Geometry check sheet. Reference: the model listing, model coordinates, mm. Face numbers are marked on the shaded views. A direction names the side the tool comes from. Give positions to 0.01 mm unless a question says otherwise; leave off trailing zeros. Write each loop counter-clockwise with the first axis right and the second up, starting at its lowest first coordinate (ties: lowest second). Pieces come first, ordered by that corner, then holes. Notation, with made-up numbers: M -8.75,25.5 L -3.75,25.5 A21 cw -3.75,40.5 Z; hole C 69.5,-16.5 d9. An arc over 180 degrees is marked long. One line per item, written item: value. Start each with the question number.
1. Gauge pin test, flat ends, axial feed: pin 1 (1.5 mm diameter, centred on x = 3.5, z = 2.5, fed in from -Y); pin 2 (0.8 mm diameter, centred on x = 16, y = 38.5, fed in from +Z); pin 3 (5 mm diameter, centred on x = 9.5, z = 4.5, fed in from -Y); pin 4 (1 mm diameter, centred on x = 8.5, z = 5, fed in from -Y). Record the tip position at first contact, or that the pin passes through.
2. Scan lines: line 1 (X direction, y = 23, z = 5.25); line 2 (Z direction, x = 24.75, y = 4.5); line 3 (Y direction, x = 8.25, z = 7.75). Record each from-to range of solid material in increasing order.
3. Release check for a two-part mould opening along Y. For the marked faces 3, 4 and 5 record: pulls with the +Y half, pulls with the -Y half, needs draft (parallel to the pull), parting line crosses it, or undercut.
4. Cross-section at A-A on x = 17.75. Record the cut outline in (y, z), then the cut area to 3 significant figures.
5. Cross-section at D-D on y = 19. Record the cut outline in (x, z), then the cut area to 3 significant figures.
6. Cross-section at B-B on y = 7.5. Record the cut outline in (x, z), then the cut area to 3 significant figures.
7. Tool access check on the marked faces 1 and 2. Record the directions out of +Z, -Z, +X, -X, +Y, -Y that give a thin tool (end or side, any length) a straight path to the whole face; none if there is none.
8. Cross-section at C-C on z = 3.75. Record the cut outline in (x, y), then the cut area to 3 significant figures.
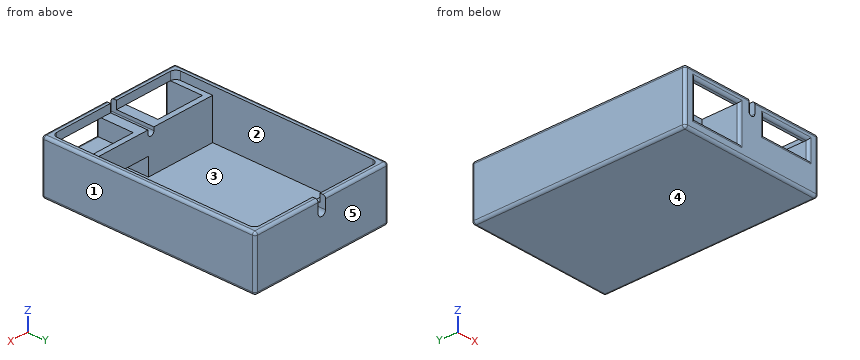
from build123d import *

# Parameters (mm, degrees)
SKETCH_2_W           = 27
SKETCH_2_H           = 40
EXTRUDE_1_DEPTH      = 10
CUT_EXTRUDE_1_DEPTH  = 1.5
CUT_EXTRUDE_2_DEPTH  = 7.5
SKETCH_9_W           = 9
SKETCH_9_H           = 4.718038217
CUT_EXTRUDE_8_DEPTH  = 3.2
SKETCH_9_3_W         = 9
SKETCH_9_3_H         = 4.718038217
CUT_EXTRUDE_9_DEPTH  = 6.5
SKETCH_12_W          = 12
SKETCH_12_H          = 3.3
CUT_EXTRUDE_10_DEPTH = 7
SKETCH_13_W          = 9
SKETCH_13_H          = 6.5
SKETCH_13_H_2        = 3.2
CUT_EXTRUDE_11_DEPTH = 3.281961783
CUT_EXTRUDE_12_REACH = 42
SKETCH_14_W          = 1.2
SKETCH_14_H          = 2.1
SKETCH_16_2_W        = 7
SKETCH_16_2_H        = 2.5
EXTRUDE_3_DEPTH      = 1
SKETCH_16_W          = 7
SKETCH_16_H          = 2.5
EXTRUDE_2_DEPTH      = 1
CUT_EXTRUDE_14_DEPTH = 2
FILLET_1_R           = 0.5


with BuildPart() as part:
    # Sketch 2 → Extrude 1 (new body)
    with BuildSketch(Plane.XY):
        with Locations((13.5, 20)):
            Rectangle(SKETCH_2_W, SKETCH_2_H)
    extrude(amount=EXTRUDE_1_DEPTH)

    # Sketch 3 → Cut-Extrude 1 (cut)
    with BuildSketch(Plane.XY.offset(10)):
        with BuildLine():
            Line((1, 38), (1, 2))
            ThreePointArc((1, 2), (1.292893219, 1.292893219), (2, 1))
            Line((2, 1), (25, 1))
            ThreePointArc((25, 1), (25.707106781, 1.292893219), (26, 2))
            Line((26, 2), (26, 38))
            ThreePointArc((26, 38), (25.707106781, 38.707106781), (25, 39))
            Line((25, 39), (2, 39))
            ThreePointArc((2, 39), (1.292893219, 38.707106781), (1, 38))
        make_face()
    extrude(amount=-CUT_EXTRUDE_1_DEPTH, mode=Mode.SUBTRACT)

    # Sketch 5 → Cut-Extrude 2 (cut)
    with BuildSketch(Plane.XY.offset(8.5)):
        with BuildLine():
            Line((2, 39), (25, 39))
            ThreePointArc((25, 39), (25.707106781, 38.707106781), (26, 38))
            Line((26, 38), (26, 8))
            Line((26, 8), (1, 8))
            Line((1, 8), (1, 38))
            ThreePointArc((1, 38), (1.292893219, 38.707106781), (2, 39))
        make_face()
    extrude(amount=-CUT_EXTRUDE_2_DEPTH, mode=Mode.SUBTRACT)

    # Sketch 9 → Cut-Extrude 8 (cut)
    with BuildSketch(Plane.XY.offset(8.5)):
        with Locations((20.5, 4.640980891)):
            Rectangle(SKETCH_9_W, SKETCH_9_H)
    extrude(amount=-CUT_EXTRUDE_8_DEPTH, mode=Mode.SUBTRACT)

    # Sketch 9_3 → Cut-Extrude 9 (cut)
    with BuildSketch(Plane.XY.offset(8.5)):
        with Locations((6.5, 4.640980891)):
            Rectangle(SKETCH_9_3_W, SKETCH_9_3_H)
    extrude(amount=-CUT_EXTRUDE_9_DEPTH, mode=Mode.SUBTRACT)

    # Sketch 12 → Cut-Extrude 10 (cut)
    with BuildSketch(Plane(origin=(0, 8, 0), x_dir=(1, 0, 0), z_dir=(0, 1, 0))):
        with Locations((20, -2.65)):
            Rectangle(SKETCH_12_W, SKETCH_12_H)
    extrude(amount=-CUT_EXTRUDE_10_DEPTH, mode=Mode.SUBTRACT)

    # Sketch 13 → Cut-Extrude 11 (cut, through all)
    with BuildSketch(Plane(origin=(0, 2.281961783, 0), x_dir=(1, 0, 0), z_dir=(0, 1, 0))):
        with Locations((6.5, -5.25)):
            Rectangle(SKETCH_13_W, SKETCH_13_H)
        with Locations((20.5, -6.9)):
            Rectangle(SKETCH_13_W, SKETCH_13_H_2)
    extrude(amount=-CUT_EXTRUDE_11_DEPTH, mode=Mode.SUBTRACT)

    # Sketch 14 → Cut-Extrude 12 (cut, up to next)
    with BuildSketch(Plane.XZ, mode=Mode.PRIVATE) as cut_extrude_12_sk1:
        with BuildLine():
            Line((12.9, 7.9), (14.1, 7.9))
            ThreePointArc((14.1, 7.9), (13.5, 7.3), (12.9, 7.9))
        make_face()
    cut_extrude_12_tool1 = extrude(cut_extrude_12_sk1.sketch, amount=-CUT_EXTRUDE_12_REACH, mode=Mode.PRIVATE) & part.part
    add(cut_extrude_12_tool1.solids().sort_by_distance((13.5, 0, 7.645352))[0], mode=Mode.SUBTRACT)
    # Sketch 14 → Cut-Extrude 12 (cut, up to next)
    with BuildSketch(Plane.XZ, mode=Mode.PRIVATE) as cut_extrude_12_sk2:
        with Locations((13.5, 8.95)):
            Rectangle(SKETCH_14_W, SKETCH_14_H)
    cut_extrude_12_tool2 = extrude(cut_extrude_12_sk2.sketch, amount=-CUT_EXTRUDE_12_REACH, mode=Mode.PRIVATE) & part.part
    add(cut_extrude_12_tool2.solids().sort_by_distance((13.5, 0, 8.95))[0], mode=Mode.SUBTRACT)

    # Sketch 16_2 → Extrude 3 (add)
    with BuildSketch(Plane.XZ.offset(-39)):
        with Locations((13.5, 7.25)):
            Rectangle(SKETCH_16_2_W, SKETCH_16_2_H)
    extrude(amount=EXTRUDE_3_DEPTH)

    # Sketch 16 → Extrude 2 (add)
    with BuildSketch(Plane.XZ.offset(-39)):
        with Locations((13.5, 7.25)):
            Rectangle(SKETCH_16_W, SKETCH_16_H)
    extrude(amount=EXTRUDE_2_DEPTH)

    # Sketch 17 → Cut-Extrude 14 (cut)
    with BuildSketch(Plane(origin=(0, 40, 0), x_dir=(1, 0, 0), z_dir=(0, 1, 0))):
        with BuildLine():
            Line((14.25, -7.75), (14.25, -10))
            Line((14.25, -10), (12.75, -10))
            Line((12.75, -10), (12.75, -7.75))
            ThreePointArc((12.75, -7.75), (13.5, -7), (14.25, -7.75))
        make_face()
    extrude(amount=-CUT_EXTRUDE_14_DEPTH, mode=Mode.SUBTRACT)

    # Fillet 1
    fillet_1_edges = [part.edges().sort_by_distance(p)[0] for p in [
        (27, 20, 10),
        (20.5, 0, 8.5),
        (25, 0, 6.9),
        (16, 0, 6.9),
        (20.5, 0, 5.3),
        (20.625, 40, 10),
        (20.55, 0, 10),
        (6.375, 40, 10),
        (0, 20, 10),
        (13.5, 40, 0),
        (27, 20, 0),
        (13.5, 0, 0),
        (0, 20, 0),
        (6.45, 0, 10),
        (0, 40, 5),
        (27, 40, 5),
        (27, 0, 5),
        (0, 0, 5),
        (6.5, 0, 8.5),
        (11, 0, 5.25),
        (2, 0, 5.25),
        (6.5, 0, 2),
    ]]
    fillet(fillet_1_edges, radius=FILLET_1_R)


solid = part.part
Report:
1. pin 1: stops at y = 0.07
1. pin 2: stops at z = 8.5
1. pin 3: stops at y = 0
1. pin 4: stops at y = 7
2. line 1: x = 0 to 1, 26 to 27
2. line 2: z = 0 to 1, 4.3 to 5.3
2. line 3: y = 7 to 8, 39 to 40
3. face 3: undercut
3. face 4: needs draft
3. face 5: pulls with the +Y half
4. outline: M 0,0.5 A0.5 ccw 0.5,0 L 39.5,0 A0.5 ccw 40,0.5 L 40,9.5 A0.5 ccw 39.5,10 L 39,10 L 39,1 L 1,1 L 1,4.3 L 8,4.3 L 8,8.5 L 7,8.5 L 7,5.3 L 0.5,5.3 A0.5 ccw 0,4.8 Z; M 0,9 A0.5 ccw 0.5,8.5 L 1,8.5 L 1,10 L 0.5,10 A0.5 ccw 0,9.5 Z
4. area: 64.7 mm^2
5. outline: M 0,0.5 A0.5 ccw 0.5,0 L 26.5,0 A0.5 ccw 27,0.5 L 27,9.5 A0.5 ccw 26.5,10 L 26,10 L 26,1 L 1,1 L 1,10 L 0.5,10 A0.5 ccw 0,9.5 Z
5. area: 44.8 mm^2
6. outline: M 0,0.5 A0.5 ccw 0.5,0 L 26.5,0 A0.5 ccw 27,0.5 L 27,9.5 A0.5 ccw 26.5,10 L 26,10 L 26,8.5 L 14.1,8.5 L 14.1,7.9 A0.6 cw 12.9,7.9 L 12.9,8.5 L 1,8.5 L 1,10 L 0.5,10 A0.5 ccw 0,9.5 Z; hole M 14,1 L 26,1 L 26,4.3 L 14,4.3 Z
6. area: 191 mm^2
7. face 1: +Z, -Z, +X, +Y, -Y
7. face 2: +Z
8. outline: M 0,0.5 A0.5 ccw 0.5,0 L 1.5,0 A0.5 ccw 2,0.5 L 2,7 L 11,7 L 11,0.5 A0.5 ccw 11.5,0 L 26.5,0 A0.5 ccw 27,0.5 L 27,39.5 A0.5 ccw 26.5,40 L 0.5,40 A0.5 ccw 0,39.5 Z; hole M 1,8 L 14,8 L 14,1 L 26,1 L 26,38 A1 ccw 25,39 L 2,39 A1 ccw 1,38 Z
8. area: 158 mm^2
